```python
from build123d import *

# Parameters (mm, degrees)
SKETCH1_W           = 34
SKETCH1_H           = 6
BOSS_EXTRUDE1_DEPTH = 5
SKETCH2_W           = 34
SKETCH2_H           = 3
BOSS_EXTRUDE2_DEPTH = 92
BOSS_EXTRUDE3_DEPTH = 3
SKETCH4_W           = 5.001426655
SKETCH4_H           = 6
BOSS_EXTRUDE4_DEPTH = 3


with BuildPart() as part:
    # Sketch1 → Boss-Extrude1 (new body)
    with BuildSketch(Plane.XY):
        with Locations((-23.102564103, 9.466666667)):
            Rectangle(SKETCH1_W, SKETCH1_H)
    extrude(amount=-BOSS_EXTRUDE1_DEPTH)

    # Sketch2 → Boss-Extrude2 (add)
    with BuildSketch(Plane(origin=(0, 0, -5), x_dir=(-1, 0, 0), z_dir=(0, 0, -1))):
        with Locations((23.102564103, 7.966666667)):
            Rectangle(SKETCH2_W, SKETCH2_H)
    extrude(amount=BOSS_EXTRUDE2_DEPTH)

    # Sketch3 → Boss-Extrude3 (add)
    with BuildSketch(Plane.ZY.offset(40.102564103)):
        Polygon((-5, 9.466666667), (-5, 6.466666667), (0, 6.466666667), (0, 12.466666667), (-5, 12.466666667), align=None)
    extrude(amount=BOSS_EXTRUDE3_DEPTH)

    # Sketch4 → Boss-Extrude4 (add)
    with BuildSketch(Plane(origin=(-6.102564103, 0, 0), x_dir=(0, 0, -1), z_dir=(1, 0, 0))):
        with Locations((2.500713328, 9.466666667)):
            Rectangle(SKETCH4_W, SKETCH4_H)
    extrude(amount=BOSS_EXTRUDE4_DEPTH)


solid = part.part
```
Read the model definition and answer for the solid it produces. Units are mm, in the model's axes. A direction names the side the tool comes from. Coordinates: 2 decimals unless noted, no trailing zeros. Loops run counter-clockwise (first coordinate to the right, second up) from the corner with the lowest first, then second, coordinate; pieces in that order, holes last.
(1) The part is cut by section C-C (z = -91). Determine the outline of the cut face in (x, y), and give its area (3 significant figures).
Solution:
outline: (-40.1, 6.47) - (-6.1, 6.47) - (-6.1, 9.47) - (-40.1, 9.47) - close
area: 102 mm2
(2) Consider line 1 along Y through (x, z) = (-15, -59); line 2 along Z through (x, y) = (-36, 11.05); line 3 along X through (y, z) = (7.5, -17). Determine where each line is inside the solid, lowest interval first.
Solution:
line 1: y = 6.47 to 9.47
line 2: z = -5 to 0
line 3: x = -40.1 to -6.1
(3) A tool of negligible diameter and unlimited length cuts with its end or side. For faces 1 (the face through (-3.103, 10, -2)), 2 (the face through (-40.103, 8, -50)), 3 (the face through (-23, 9.467, -50)), 4 (the face through (-5, 9, -5.001)), from which of +Z, -Z, +X, -X, +Y, -Y can it reach the whole face along a straight path? Write none if from no direction.
Solution:
face 1: +Z, -Z, +X, +Y, -Y
face 2: -Z, -X, +Y, -Y
face 3: -Z, +X, -X, +Y
face 4: -Z, +X, +Y, -Y
(4) Flat-ended cylindrical pins translate along their axes: pin 1 Ø2.5 at (y, z) = (7.5, -43.5) entering from +X; pin 2 Ø1.8 at (x, y) = (-32, 10.5) entering from -Z; pin 3 Ø8 at (x, z) = (-10, -39.5) entering from +Y. Find the tip coordinate at first contact, or state that the pin passes through.
Solution:
pin 1: stops at x = -6.1
pin 2: stops at z = -5
pin 3: stops at y = 9.47
(5) The part is cut by section A-A (y = 7.55). Determine the outline of the cut face in (x, z), and give its area (3 significant figures).
Solution:
outline: (-43.1, -5) - (-40.1, -5) - (-40.1, -97) - (-6.1, -97) - (-6.1, -5) - (-3.1, -5) - (-3.1, 0) - (-43.1, 0) - close
area: 3,330 mm2
(6) The part is cut by section B-B (x = -28). Determine the outline of the cut face in (y, z).
Solution:
outline: (6.47, -97) - (9.47, -97) - (9.47, -5) - (12.47, -5) - (12.47, 0) - (6.47, 0) - close
